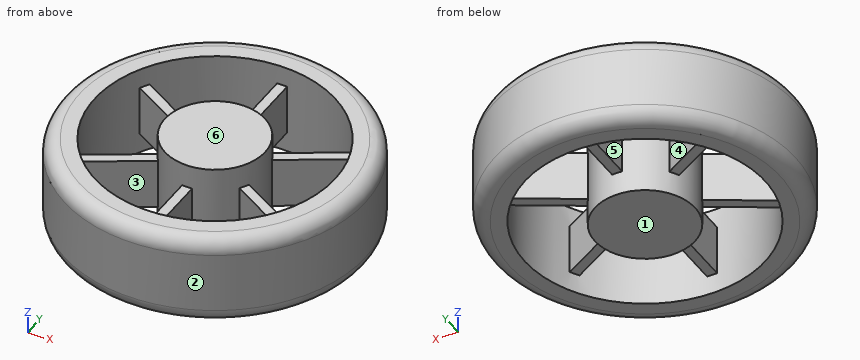
from build123d import *

# Parameters (mm, degrees)
SKETCH1_R           = 50
BOSS_EXTRUDE1_DEPTH = 48.5
SKETCH2_R           = 150
SKETCH2_R_2         = 120
BOSS_EXTRUDE2_DEPTH = 45
BOSS_EXTRUDE3_DEPTH = 25
CIRPATTERN15_COUNT  = 6
FILLET1_R           = 15


with BuildPart() as part:
    # Sketch1 → Boss-Extrude1 (new body, symmetric)
    with BuildSketch(Plane.XY):
        Circle(SKETCH1_R)
    extrude(amount=BOSS_EXTRUDE1_DEPTH, both=True)



with BuildPart() as body_2:
    # Sketch2 → Boss-Extrude2 (new body, symmetric)
    with BuildSketch(Plane.XY):
        Circle(SKETCH2_R)
        Circle(SKETCH2_R_2, mode=Mode.SUBTRACT)
    extrude(amount=BOSS_EXTRUDE2_DEPTH, both=True)


with BuildPart() as part_1:
    add(part.part)

    add(body_2.part)  # Boss-Extrude3 merges body 2
    # Sketch3 → Boss-Extrude3 (add, symmetric)
    with BuildSketch(Plane.XY):
        with BuildLine():
            Line((-5, 119.895788083), (-5, 49.749371855))
            ThreePointArc((-5, 49.749371855), (0, 50), (5, 49.749371855))
            Line((5, 49.749371855), (5, 119.895788083))
            ThreePointArc((5, 119.895788083), (0, 120), (-5, 119.895788083))
        make_face()
    boss_extrude3 = extrude(amount=BOSS_EXTRUDE3_DEPTH, both=True)

    # CirPattern15: Boss-Extrude3 ×6 about axis
    cirpattern15_axis = Axis((0, 0, 0), (0, 0, 1))
    for i in range(1, CIRPATTERN15_COUNT):
        add(boss_extrude3.rotate(cirpattern15_axis, i * 360 / CIRPATTERN15_COUNT))

    # Fillet1
    fillet1_edges = [part_1.edges().sort_by_distance(p)[0] for p in [
        (-150, 0, 45),
        (-150, 0, -45),
    ]]
    fillet(fillet1_edges, radius=FILLET1_R)


solid = part_1.part
Verification items for the finished model (mm, model axes). Face numbers are marked on the shaded views. A direction names the side the tool comes from. Coordinates: 2 decimals unless noted, no trailing zeros. Order: outer loops, then holes, each group sorted by start corner. A loop starts at its lowest first (then second) coordinate and runs counter-clockwise, first axis right, second up. Notation, with made-up numbers: M 82.25,48 L 129.25,48 A16 ccw 129.25,68 Z; hole C 21.5,59.25 d4. An arc over 180 degrees is marked long. One line per item, written item: value. Start each with the question number.
Item 1: Sectioned sample at C-C (x = 0). Enter the section's corners in (y, z).
Item 2: Sectioned sample at A-A (y = 0). Enter the section's corners in (x, z), then the cut area to 3 significant figures.
Item 3: Sectioned sample at B-B (z = 5.5). Enter the section's corners in (x, y), then the cut area to 3 significant figures.
Item 4: Sectioned sample at D-D (z = -41.5). Enter the section's corners in (x, y).
Item 5: Scan lines: probe 1 along X at (y, z) = (14, 18); probe 2 along X at (y, z) = (64.5, -5); probe 3 along Y at (x, z) = (20, -21). Record each from-to range of solid material in increasing order.
Item 6: Mould release check, pull along Y, two halves, no side actions. Record for the marked faces 1, 2, 3 and 4: released by +Y, released by -Y, zero draft, split by the parting line, or undercut.
Item 7: Access from +Z, -Z, +X, -X, +Y, -Y to the whole of each face (thin tool, end or side, straight path). Record for the marked faces 5 and 6.
Item 8: Gauge pin test, flat ends, axial feed: pin 1 (6 mm diameter, centred on x = 59.5, z = -19, fed in from -Y); pin 2 (4 mm diameter, centred on x = -95, y = -54, fed in from -Z); pin 3 (5 mm diameter, centred on x = 77.5, y = -95.5, fed in from -Z). Record the tip position at first contact, or that the pin passes through.
Conclusion:
1. outline: M -150,-30 A15 ccw -135,-45 L -120,-45 L -120,-25 L -50,-25 L -50,-48.5 L 50,-48.5 L 50,-25 L 120,-25 L 120,-45 L 135,-45 A15 ccw 150,-30 L 150,30 A15 ccw 135,45 L 120,45 L 120,25 L 50,25 L 50,48.5 L -50,48.5 L -50,25 L -120,25 L -120,45 L -135,45 A15 ccw -150,30 Z
2. outline: M -150,-30 A15 ccw -135,-45 L -120,-45 L -120,45 L -135,45 A15 ccw -150,30 Z; M -50,-48.5 L 50,-48.5 L 50,48.5 L -50,48.5 Z; M 120,-45 L 135,-45 A15 ccw 150,-30 L 150,30 A15 ccw 135,45 L 120,45 Z
2. area: 14,900 mm^2
3. outline: C 0,0 d300; hole M -106.33,-55.62 L -45.58,-20.54 A50 cw -45.58,20.54 L -106.33,55.62 A120 ccw Z; hole M -101.33,-64.28 A120 ccw -5,-119.9 L -5,-49.75 A50 cw -40.58,-29.2 Z; hole M -101.33,64.28 L -40.58,29.2 A50 cw -5,49.75 L -5,119.9 A120 ccw Z; hole M 5,-119.9 A120 ccw 101.33,-64.28 L 40.58,-29.2 A50 cw 5,-49.75 Z; hole M 5,49.75 A50 cw 40.58,29.2 L 101.33,64.28 A120 ccw 5,119.9 Z; hole M 45.58,-20.54 L 106.33,-55.62 A120 ccw 106.33,55.62 L 45.58,20.54 A50 cw Z
3. area: 37,500 mm^2
4. outline: C 0,0 d289.26; C 0,0 d100; hole C 0,0 d240
5. probe 1: x = -149.35 to -119.18, -48 to 48, 119.18 to 149.35
5. probe 2: x = -135.42 to -101.19, -5 to 5, 101.19 to 135.42
5. probe 3: y = -148.66 to -118.32, -45.83 to 45.83, 118.32 to 148.66
6. face 1: zero draft
6. face 2: split by the parting line
6. face 3: undercut
6. face 4: undercut
7. face 5: +Z, -Z
7. face 6: +Z, +X, -X, +Y, -Y
8. pin 1: stops at y = -138.95
8. pin 2: stops at z = -25
8. pin 3: stops at z = -45
